from build123d import *

# Parameters (mm, degrees)
SKETCH1_W               = 25.4
SKETCH1_H               = 8.001
BOSS_EXTRUDE1_DEPTH     = 6.35
CUT_EXTRUDE1_DEPTH      = 25.4
CUT_EXTRUDE2_DEPTH      = 14.940238753
CUT_EXTRUDE2_DEPTH_BACK = 1.905
CUT_EXTRUDE3_START      = -25.4
SKETCH5_R               = 0.9271
CUT_EXTRUDE3_DEPTH      = 6.35
SKETCH6_W               = 10.795
SKETCH6_H               = 8.001
CUT_EXTRUDE4_DEPTH      = 0.508
CHAMFER1_SIZE           = 2.54


with BuildPart() as part:
    # Sketch1 → Boss-Extrude1 (new body)
    with BuildSketch(Plane(origin=(0, 0, 0), x_dir=(1, 0, 0), z_dir=(0, 1, 0))):
        Rectangle(SKETCH1_W, SKETCH1_H)
    extrude(amount=BOSS_EXTRUDE1_DEPTH)

    # Sketch2 → Cut-Extrude1 (cut)
    with BuildSketch(Plane(origin=(0, 0, -4.0005), x_dir=(-1, 0, 0), z_dir=(0, 0, -1))):
        with BuildLine():
            Line((5.3975, 4.1275), (-5.3975, 4.1275))
            ThreePointArc((-5.3975, 4.1275), (-7.62, 6.35), (-5.3975, 8.5725))
            Line((-5.3975, 8.5725), (5.3975, 8.5725))
            ThreePointArc((5.3975, 8.5725), (7.62, 6.35), (5.3975, 4.1275))
        make_face()
    extrude(amount=-CUT_EXTRUDE1_DEPTH, mode=Mode.SUBTRACT)

    # Sketch4 → Cut-Extrude2 (cut, two sides: drawn at the far end of the back side and taken through both)
    with BuildSketch(Plane(origin=(0, 4.1275, 0), x_dir=(1, 0, 0), z_dir=(0, 1, 0)).offset(-CUT_EXTRUDE2_DEPTH_BACK)):
        with BuildLine():
            Line((0.8255, -4.0005), (-0.9525, -4.0005))
            ThreePointArc((-0.9525, -4.0005), (-2.254410358, -0.857410358), (-5.3975, 0.4445))
            Line((-5.3975, 0.4445), (-7.185501788, 0.4445))
            ThreePointArc((-7.185501788, 0.4445), (-7.769218436, 0.686283352), (-8.011001788, 1.27))
            Line((-8.011001788, 1.27), (-8.011001788, 1.397))
            ThreePointArc((-8.011001788, 1.397), (-7.769218436, 1.980716648), (-7.185501788, 2.2225))
            Line((-7.185501788, 2.2225), (-5.3975, 2.2225))
            ThreePointArc((-5.3975, 2.2225), (-0.997174501, 0.399825499), (0.8255, -4.0005))
        make_face()
    extrude(amount=CUT_EXTRUDE2_DEPTH + CUT_EXTRUDE2_DEPTH_BACK, mode=Mode.SUBTRACT)

    # Sketch5 → Cut-Extrude3 (cut)
    with BuildSketch(Plane(origin=(12.7, 0, 0), x_dir=(0, 0, -1), z_dir=(1, 0, 0)).offset(CUT_EXTRUDE3_START)):
        with Locations(Location((1.3335, 3.81, 0), (0, 0, 180))):
            Circle(SKETCH5_R)
    extrude(amount=CUT_EXTRUDE3_DEPTH, mode=Mode.SUBTRACT)

    # Sketch6 → Cut-Extrude4 (cut)
    with BuildSketch(Plane(origin=(0, 4.1275, 0), x_dir=(1, 0, 0), z_dir=(0, 1, 0))):
        Rectangle(SKETCH6_W, SKETCH6_H)
    extrude(amount=-CUT_EXTRUDE4_DEPTH, mode=Mode.SUBTRACT)

    # Chamfer1
    chamfer1_edges = [part.edges().sort_by_distance(p)[0] for p in [
        (-12.7, 0, 0),
        (12.7, 0, 0),
    ]]
    chamfer(chamfer1_edges, length=CHAMFER1_SIZE)


solid = part.part
Source: CAD feature listing. Evaluate the final solid. Frame: model axes, mm. A direction names the side the tool comes from. Coordinates: 2 decimals unless noted, no trailing zeros. Order: outer loops, then holes, each group sorted by start corner. A loop starts at its lowest first (then second) coordinate and runs counter-clockwise, first axis right, second up. Notation, with made-up numbers: M -25,-21 L -1,-21 A18 cw -1,-9 Z; hole C -25.75,68 d4. An arc over 180 degrees is marked long. Write each question's results on one line, items separated by ' | '. Start each with the question number.
1. Material intervals for L1, parallel to Z at x = -9, y = 3.81; L2, parallel to Y at x = -5.5, z = -3; L3, parallel to Y at x = 3.75, z = 2.5, sorted ascending.
2. Reachability of faces 4 (the face through (6.95, 4.76, -0.06)), 5 (the face through (-3, 2.222, 0)), 6 (the face through (-10.28, 3.77, -2.26)) from +Z, -Z, +X, -X, +Y, -Y: full face, straight path, thin tool, end or side. Return the list, or none.
3. Section A-A, the plane y = 5.5. Return the cut outline in (x, z), then the cut area to 3 significant figures.
4. Section D-D, the plane y = 1.5. Return the cut outline in (x, z), then the cut area to 3 significant figures.
5. Section B-B, the plane x = -3.25. Return the cut outline in (y, z), then the cut area to 3 significant figures.
6. Pin query (flat end, axial travel): pin 1 (2 mm diameter, centred on x = 0, z = 0.5, fed in from +Y); pin 2 (1 mm diameter, centred on x = -3.5, y = 5.5, fed in from +Z). Return the tip coordinate at first contact, or that it passes through.
7. Draft query along X for faces 1 (the face through (-1, 2.9, -0.4)), 2 (the face through (0, 2, -4)), 3 (the face through (-11.41, 1.25, 0.06)). Return one class per face: +X half, -X half, draft (parallel to the pull), parting line (faces both ways), or undercut.
Solution:
1) L1: -4 to -2.26, -0.41 to 4 | L2: 0 to 4.13 | L3: 0 to 3.62
2) face 4: +Z, -Z, +Y | face 5: +Y | face 6: -X
3) outline: M -12.7,-4 L -7.45,-4 L -7.45,-2.18 A0.83 cw -8.01,-1.4 L -8.01,-1.27 A0.83 cw -7.45,-0.49 L -7.45,4 L -12.7,4 Z; M 7.45,-4 L 12.7,-4 L 12.7,4 L 7.45,4 Z | area: 83.3 mm²
4) outline: M -11.66,-4 L 11.66,-4 L 11.66,4 L -11.66,4 Z | area: 187 mm²
5) outline: M 0,-4 L 3.62,-4 L 3.62,-1.84 L 2.22,-1.84 L 2.22,0.11 L 3.62,0.11 L 3.62,4 L 0,4 Z | area: 26.2 mm²
6) pin 1: y = 3.62 | pin 2: through
7) face 1: undercut | face 2: draft | face 3: -X half
